from build123d import *

# Parameters (mm, degrees)
F0_R     = 27.5956860517
F1_DEPTH = 2
F0_R_2   = 35
F2_DEPTH = 4


with BuildPart() as f1:
    # F0 (on Top) → F1 (new body)
    with BuildSketch(Plane.XY):
        Circle(F0_R)
        Polygon((-9.6259148038, 1.1057544772), (-15.0088759263, -10.9735011217), (-15.5956118662, -10.9735011217), (-20.8694128139, 1.1057544772), (-20.8694128139, -9.9057781613), (-18.952287243, -10.1957348758), (-18.952287243, -10.9735011217), (-24.0384691402, -10.9735011217), (-24.0384691402, -10.1957348758), (-22.2032137004, -9.9057781613), (-22.2032137004, 2.265581335), (-24.0384691402, 2.5453042831), (-24.0384691402, 3.3230705289), (-18.4201313906, 3.3230705289), (-14.3368585999, -6.0817607859), (-10.1683044226, 3.3230705289), (-4.4339839872, 3.3230705289), (-4.4339839872, 2.5453042831), (-6.2658281715, 2.265581335), (-6.2658281715, -9.9057781613), (-4.4339839872, -10.1957348758), (-4.4339839872, -10.9735011217), (-11.5430403747, -10.9735011217), (-11.5430403747, -10.1957348758), (-9.6259148038, -9.9057781613), align=None, mode=Mode.SUBTRACT)
        Polygon((7.508821393, 3.3230705289), (11.7183106359, 3.3230705289), (11.7183106359, 2.5453042831), (10.3640422166, 2.2553475686), (4.84121962, -11.3043929017), (3.4255486024, -11.3043929017), (-2.3838194532, 2.2553475686), (-3.5572913329, 2.5453042831), (-3.5572913329, 3.3230705289), (2.6580161229, 3.3230705289), (2.6580161229, 2.5453042831), (1.174119996, 2.2553475686), (5.1959901883, -7.1153711916), (8.948371199, 2.2553475686), (7.508821393, 2.5453042831), align=None, mode=Mode.SUBTRACT)
        with BuildLine():
            Line((19.4584492842, -5.3653971385), (17.5379124579, -5.3653971385))
            Line((17.5379124579, -5.3653971385), (17.5379124579, -9.9057781613))
            Line((17.5379124579, -9.9057781613), (19.9155575165, -10.1957348758))
            Line((19.9155575165, -10.1957348758), (19.9155575165, -10.9735011217))
            Line((19.9155575165, -10.9735011217), (12.475609349, -10.9735011217))
            Line((12.475609349, -10.9735011217), (12.475609349, -10.1957348758))
            Line((12.475609349, -10.1957348758), (14.1710033147, -9.9057781613))
            Line((14.1710033147, -9.9057781613), (14.1710033147, 2.265581335))
            Line((14.1710033147, 2.265581335), (12.3357478749, 2.5453042831))
            Line((12.3357478749, 2.5453042831), (12.3357478749, 3.3230705289))
            Line((12.3357478749, 3.3230705289), (18.6363367174, 3.3230705289))
            add(Edge.make_bspline(
                [(18.6363367174, 3.3230705289), (21.675765336, 3.3230705289), (23.178423368, 2.3048107729)],
                knots=[0, 0, 0, 1, 1, 1], degree=2))
            add(Edge.make_bspline(
                [(23.178423368, 2.3048107729), (24.6810814, 1.2865510168), (24.6810814, -0.8898299694)],
                knots=[0, 0, 0, 1, 1, 1], degree=2))
            add(Edge.make_bspline(
                [(24.6810814, -0.8898299694), (24.6810814, -5.3653971385), (19.4584492842, -5.3653971385)],
                knots=[0, 0, 0, 1, 1, 1], degree=2))
        make_face(mode=Mode.SUBTRACT)
        Polygon((1.3197273183, 17.2339269534), (1.3197273183, 7.1216629411), (3.216591065, 6.9262442858), (3.216591065, 6.2253427091), (-2.9221602911, 6.2253427091), (-2.9221602911, 6.9262442858), (-1.0331132906, 7.1216629411), (-1.0331132906, 15.3526966991), (-2.9143435449, 14.7351737486), (-2.9143435449, 15.4256529971), (0.1628488794, 17.2339269534), align=None, mode=Mode.SUBTRACT)
    extrude(amount=F1_DEPTH)

    # F0 (on Top) → F2 (join)
    with BuildSketch(Plane.XY):
        with Locations((0.418909197, 0)):
            Circle(F0_R_2)
        Circle(F0_R, mode=Mode.SUBTRACT)
    extrude(amount=F2_DEPTH)


solid = f1.part
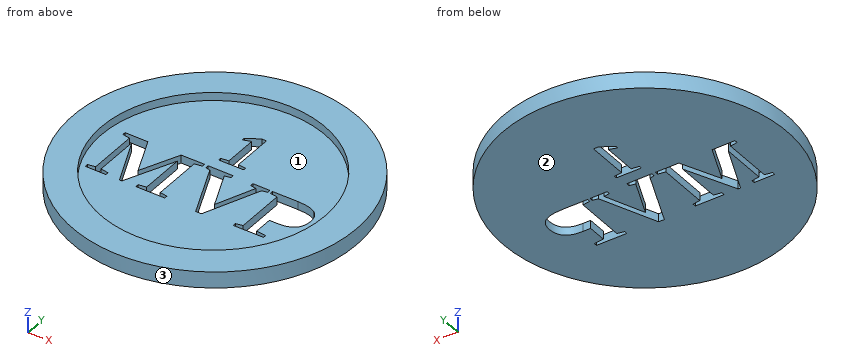
Design review of the part built by this model. Coordinates are the model's own, in mm. Face numbers are marked on the shaded views. Give positions to 0.01 mm unless a question says otherwise; leave off trailing zeros. Loops run counter-clockwise (first coordinate to the right, second up) from the corner with the lowest first, then second, coordinate; pieces in that order, holes last. Notation, with made-up numbers: (11, 34) - (58, 34) arc R16 cw to (58, 45) - close; hole circle Ø3 at (33, -37). An arc over 180 degrees is marked (long way). Write item = value, one per line.
1) Draft analysis for pull direction Y (two halves, no side actions). For the marked faces 1, 2 and 3, state which applies: +Y half, -Y half, draft (parallel to the pull), parting line (faces both ways), or undercut.
Result sheet:
face_1 = undercut
face_2 = draft
face_3 = parting line
2) Take a section at C-C on z = 3.1. State the section outline as (x, y) points, and give its area (3 significant figures).
Result sheet:
outline = circle Ø70 at (0.42, 0); hole circle Ø55.19 at (0, 0)
area = 1,460 mm2
3) Clearance check with flat-ended pins moving along their axes: pin 1 Ø0.6 at (y, z) = (-10.5, 1) entering from -X; pin 2 Ø0.6 at (x, z) = (-8.5, 1.5) entering from +Y; pin 3 Ø5 at (x, y) = (5, 14) entering from +Z. State where each tip first meets the part, or that it passes through.
Result sheet:
pin_1 = -33.06
pin_2 = 33.92
pin_3 = 2
4) Take a section at A-A on x = -13. State the section outline as (y, z) points.
Result sheet:
outline = (-32.33, 0) - (-6.47, 0) - (-6.47, 2) - (-24.34, 2) - (-24.34, 4) - (-32.33, 4) - close; (-3.07, 0) - (32.33, 0) - (32.33, 4) - (24.34, 4) - (24.34, 2) - (-3.07, 2) - close
5) Take a section at D-D on x = -26. State the section outline as (y, z) points, and give its area (3 significant figures).
Result sheet:
outline = (-22.96, 0) - (22.96, 0) - (22.96, 4) - (9.25, 4) - (9.25, 2) - (-9.25, 2) - (-9.25, 4) - (-22.96, 4) - close
area = 147 mm2
6) To check wall thickness, follow line 1 (Y direction, x = 0, z = 3.1); line 2 (Y direction, x = 18, z = 1.4); line 3 (Y direction, x = 1, z = 0.55). State the ranges of each line that lie inside material, in increasing order.
Result sheet:
line_1 = -35 to -27.6, 27.6 to 35
line_2 = -30.26 to -10.97, -9.96 to -5.37, 3.32 to 30.26
line_3 = -35 to -5.64, 3.32 to 6.23, 17.23 to 35
7) Take a section at B-B on y = 0. Count the separate pieces of the cut face and the enclosed holes in it, and give its area (3 significant figures).
Result sheet:
separate_pieces = 8
enclosed_holes = 0
area = 120 mm2
